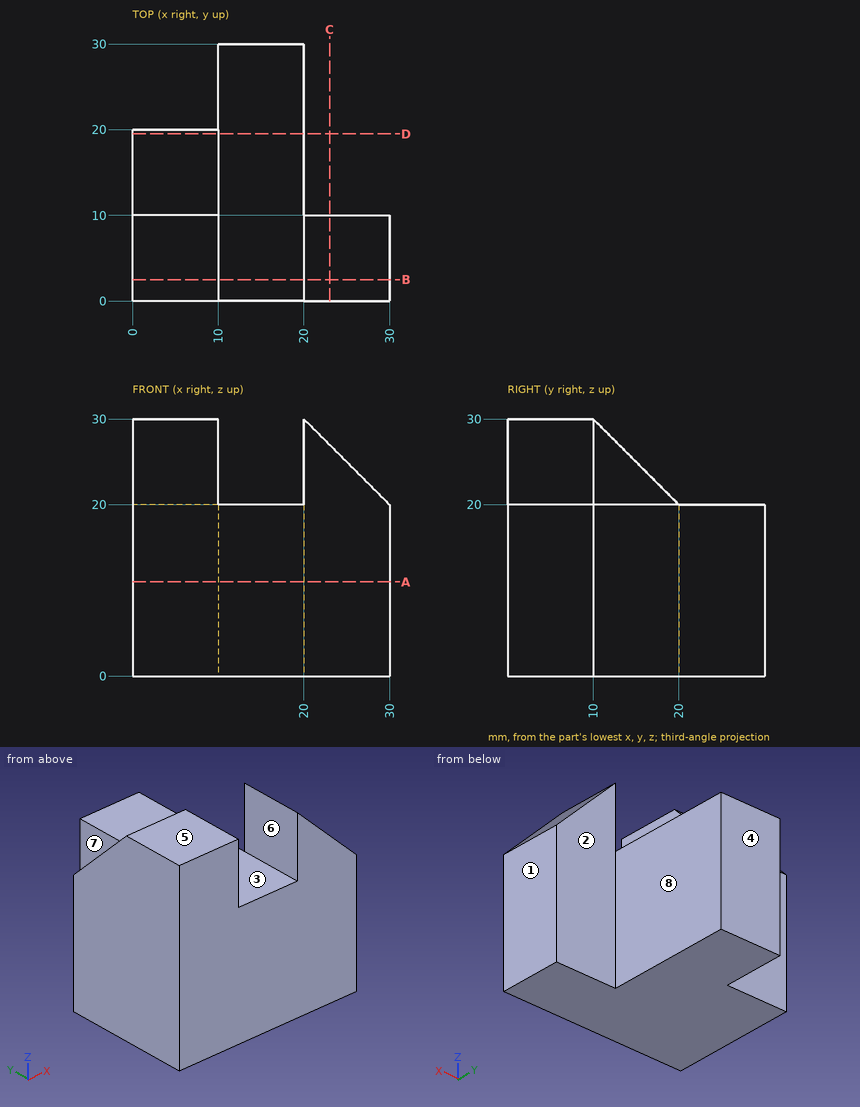
Source: three-view drawing plus pictorial views. Frame: mm from the lowest corner of the part. A direction names the side the tool comes from. Round coordinates to 2 decimals unless told otherwise and drop trailing zeros. Loops run counter-clockwise (first coordinate to the right, second up) from the corner with the lowest first, then second, coordinate; pieces in that order, holes last.
Q1. Access query for the marked faces 4, 5, 6, 7 and 8. Directions: +Z, -Z, +X, -X, +Y, -Y. A direction counts if a zero-diameter tool reaches every point of the face in a straight line with its end or side. Return the directions, or none.
Q2. Section A-A, the plane z = 11. Return loops of the section in (x, y), plus the area to 3 significant figures.
Q3. Mould query, pull axis X, two halves, no side actions, for the marked faces 1, 2 and 3. Classes: pulls with the +X half, pulls with the -X half, needs draft (parallel to the pull), parting line crosses it, or undercut.
Q4. Section D-D, the plane y = 19.5. Return loops of the section in (x, z), plus the area to 3 significant figures.
Q5. Section B-B, the plane y = 2.5. Return loops of the section in (x, z).
Q6. Ray query, line 1 (X direction, y = 8, z = 28.5); line 2 (Y direction, x = 20.5, z = 10); line 3 (Y direction, x = 2.75, z = 3). Return the intervals inside material, ascending.
Q7. First-contact query: P1, Ø10, axis at y = 21.5, z = 6, coming from the +X side; P2, Ø11, axis at x = 7, z = 13, coming from the +Y side; P3, Ø3, axis at x = 14.5, y = 14, coming from the +Z side; P4, Ø3, axis at y = 13.5, z = 23, coming from the +X side. Flat tips, straight axial feed; report the tip coordinate or a pass-through.
Q8. Section C-C, the plane x = 23. Return loops of the section in (y, z).
Solutions:
1. face 4: +Z, -Z, +X, -X, +Y
1. face 5: +Z, +X, -X, +Y, -Y
1. face 6: +Z, +Y, -Y
1. face 7: +Z, -Z, -X, +Y
1. face 8: +Z, -Z, +X, +Y
2. outline: (0, 0) - (30, 0) - (30, 10) - (20, 10) - (20, 30) - (10, 30) - (10, 20) - (0, 20) - close
2. area: 600 mm2
3. face 1: pulls with the +X half
3. face 2: needs draft
3. face 3: undercut
4. outline: (0, 0) - (20, 0) - (20, 20) - (10, 20) - (10, 20.5) - (0, 20.5) - close
4. area: 405 mm2
5. outline: (0, 0) - (30, 0) - (30, 20) - (20, 30) - (20, 20) - (10, 20) - (10, 30) - (0, 30) - close
6. line 1: x = 0 to 10, 20 to 21.5
6. line 2: y = 0 to 10
6. line 3: y = 0 to 20
7. P1: stops at x = 20
7. P2: stops at y = 30
7. P3: stops at z = 20
7. P4: stops at x = 10
8. outline: (0, 0) - (10, 0) - (10, 27) - (0, 27) - close
